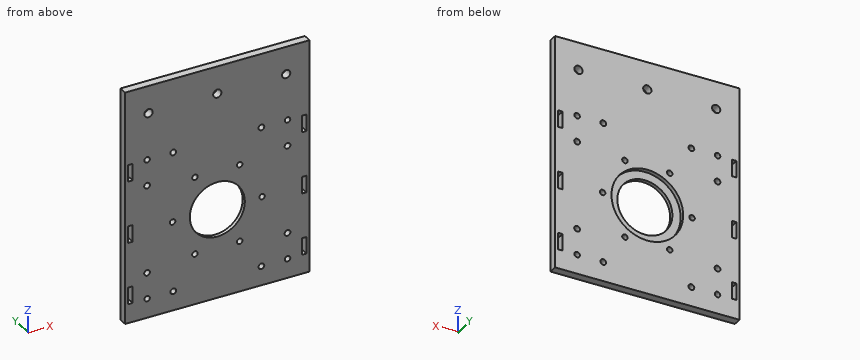
from build123d import *

# Parameters (mm, degrees)
SKETCH15_W          = 130
SKETCH15_H          = 130
SKETCH15_R          = 20
SKETCH15_R_2        = 2
BOSS_EXTRUDE1_DEPTH = 6
SKETCH16_R          = 26.05
CUT_EXTRUDE6_DEPTH  = 3.2
SKETCH17_R          = 2
CUT_EXTRUDE7_DEPTH  = 7
SKETCH18_W          = 130
SKETCH18_H          = 40
SKETCH18_R          = 3
BOSS_EXTRUDE2_DEPTH = 6
SKETCH21_W          = 2
SKETCH21_H          = 170
BOSS_EXTRUDE3_DEPTH = 6
SKETCH20_W          = 3.2
SKETCH20_H          = 12.2
CUT_EXTRUDE8_DEPTH  = 10


with BuildPart() as part:
    # Sketch15 → Boss-Extrude1 (new body)
    with BuildSketch(Plane(origin=(0, 0, 0), x_dir=(1, 0, 0), z_dir=(0, 1, 0))):
        Rectangle(SKETCH15_W, SKETCH15_H)
        Circle(SKETCH15_R, mode=Mode.SUBTRACT)
        with Locations((32.5, 0)):
            Circle(SKETCH15_R_2, mode=Mode.SUBTRACT)
        with Locations((16.25, -28.145825623)):
            Circle(SKETCH15_R_2, mode=Mode.SUBTRACT)
        with Locations((-16.25, -28.145825623)):
            Circle(SKETCH15_R_2, mode=Mode.SUBTRACT)
        with Locations((-32.5, 0)):
            Circle(SKETCH15_R_2, mode=Mode.SUBTRACT)
        with Locations((-16.25, 28.145825623)):
            Circle(SKETCH15_R_2, mode=Mode.SUBTRACT)
        with Locations((16.25, 28.145825623)):
            Circle(SKETCH15_R_2, mode=Mode.SUBTRACT)
    extrude(amount=BOSS_EXTRUDE1_DEPTH)

    # Sketch16 → Cut-Extrude6 (cut)
    with BuildSketch(Plane(origin=(0, 6, 0), x_dir=(1, 0, 0), z_dir=(0, 1, 0))):
        Circle(SKETCH16_R)
    extrude(amount=-CUT_EXTRUDE6_DEPTH, mode=Mode.SUBTRACT)

    # Sketch17 → Cut-Extrude7 (cut, through all)
    with BuildSketch(Plane.XZ):
        with Locations((-51, 51)):
            Circle(SKETCH17_R)
        with BuildLine():
            ThreePointArc((-31.999, 53.1), (-29.899, 51), (-31.999, 48.9))
            Line((-31.999, 48.9), (-32, 48.9))
            ThreePointArc((-32, 48.9), (-34.1, 51), (-32, 53.1))
            Line((-32, 53.1), (-31.999, 53.1))
        make_face()
        with BuildLine():
            Line((-53.1, 32), (-53.1, 31.999))
            ThreePointArc((-53.1, 31.999), (-51, 29.899), (-48.9, 31.999))
            Line((-48.9, 31.999), (-48.9, 32))
            ThreePointArc((-48.9, 32), (-51, 34.1), (-53.1, 32))
        make_face()
        with Locations((51, 51)):
            Circle(SKETCH17_R)
        with BuildLine():
            ThreePointArc((53.1, 31.999), (51, 29.899), (48.9, 31.999))
            Line((48.9, 31.999), (48.9, 32))
            ThreePointArc((48.9, 32), (51, 34.1), (53.1, 32))
            Line((53.1, 32), (53.1, 31.999))
        make_face()
        with Locations((51, -51)):
            Circle(SKETCH17_R)
        with BuildLine():
            Line((53.1, -32), (53.1, -31.999))
            ThreePointArc((53.1, -31.999), (51, -29.899), (48.9, -31.999))
            Line((48.9, -31.999), (48.9, -32))
            ThreePointArc((48.9, -32), (51, -34.1), (53.1, -32))
        make_face()
        with BuildLine():
            ThreePointArc((31.999, -53.1), (29.899, -51), (31.999, -48.9))
            Line((31.999, -48.9), (32, -48.9))
            ThreePointArc((32, -48.9), (34.1, -51), (32, -53.1))
            Line((32, -53.1), (31.999, -53.1))
        make_face()
        with BuildLine():
            ThreePointArc((-32, -53.1), (-34.1, -51), (-32, -48.9))
            Line((-32, -48.9), (-31.999, -48.9))
            ThreePointArc((-31.999, -48.9), (-29.899, -51), (-31.999, -53.1))
            Line((-31.999, -53.1), (-32, -53.1))
        make_face()
        with Locations((-51, -51)):
            Circle(SKETCH17_R)
        with BuildLine():
            Line((-53.1, -32), (-53.1, -31.999))
            ThreePointArc((-53.1, -31.999), (-51, -29.899), (-48.9, -31.999))
            Line((-48.9, -31.999), (-48.9, -32))
            ThreePointArc((-48.9, -32), (-51, -34.1), (-53.1, -32))
        make_face()
        with BuildLine():
            ThreePointArc((32, 53.1), (34.1, 51), (32, 48.9))
            Line((32, 48.9), (31.999, 48.9))
            ThreePointArc((31.999, 48.9), (29.899, 51), (31.999, 53.1))
            Line((31.999, 53.1), (32, 53.1))
        make_face()
    extrude(amount=-CUT_EXTRUDE7_DEPTH, mode=Mode.SUBTRACT)

    # Sketch18 → Boss-Extrude2 (add)
    with BuildSketch(Plane(origin=(0, 6, 0), x_dir=(1, 0, 0), z_dir=(0, 1, 0))):
        with Locations((0, -85)):
            Rectangle(SKETCH18_W, SKETCH18_H)
        with Locations((50, -85)):
            Circle(SKETCH18_R, mode=Mode.SUBTRACT)
        with Locations((0, -85)):
            Circle(SKETCH18_R, mode=Mode.SUBTRACT)
        with Locations((-50, -85)):
            Circle(SKETCH18_R, mode=Mode.SUBTRACT)
    extrude(amount=-BOSS_EXTRUDE2_DEPTH)

    # Sketch21 → Boss-Extrude3 (add)
    with BuildSketch(Plane(origin=(0, 6, 0), x_dir=(1, 0, 0), z_dir=(0, 1, 0))):
        with Locations((-66, -20)):
            Rectangle(SKETCH21_W, SKETCH21_H)
        with Locations((66, -20)):
            Rectangle(SKETCH21_W, SKETCH21_H)
    extrude(amount=-BOSS_EXTRUDE3_DEPTH)

    # Sketch20 → Cut-Extrude8 (cut)
    with BuildSketch(Plane(origin=(0, 6, 0), x_dir=(1, 0, 0), z_dir=(0, 1, 0))):
        with Locations((-63.1, 45)):
            Rectangle(SKETCH20_W, SKETCH20_H)
        with Locations((-63.1, 0)):
            Rectangle(SKETCH20_W, SKETCH20_H)
        with Locations((-63.1, -45)):
            Rectangle(SKETCH20_W, SKETCH20_H)
        with Locations((63.1, -45)):
            Rectangle(SKETCH20_W, SKETCH20_H)
        with Locations((63.1, 0)):
            Rectangle(SKETCH20_W, SKETCH20_H)
        with Locations((63.1, 45)):
            Rectangle(SKETCH20_W, SKETCH20_H)
    extrude(amount=-CUT_EXTRUDE8_DEPTH, mode=Mode.SUBTRACT)


solid = part.part
Could you check a few things on this model? Use its own coordinates, in mm. Coordinates: 2 decimals unless noted, no trailing zeros. Write each loop counter-clockwise with the first axis right and the second up, starting at its lowest first coordinate (ties: lowest second). Pieces come first, ordered by that corner, then holes. Notation, with made-up numbers: (18.25, -38) - (73.25, -38) arc R22 ccw to (73.25, -12) - close; hole circle Ø2 at (49, 42.25). An arc over 180 degrees is marked (long way). Write item = value, one per line.
1) Suppose I cut it at C-C on x = -16.25. Please give me the cut outline in (y, z).
Result set:
outline = (0, -65) - (6, -65) - (6, -30.15) - (0, -30.15) - close; (0, -26.15) - (6, -26.15) - (6, -20.36) - (2.8, -20.36) - (2.8, -11.66) - (0, -11.66) - close; (0, 11.66) - (2.8, 11.66) - (2.8, 20.36) - (6, 20.36) - (6, 26.15) - (0, 26.15) - close; (0, 30.15) - (6, 30.15) - (6, 105) - (0, 105) - close
2) Suppose I cut it at B-B on z = 85. Please give me the cut outline in (x, y).
Result set:
outline = (-67, 0) - (-53, 0) - (-53, 6) - (-67, 6) - close; (-47, 0) - (-3, 0) - (-3, 6) - (-47, 6) - close; (3, 0) - (47, 0) - (47, 6) - (3, 6) - close; (53, 0) - (67, 0) - (67, 6) - (53, 6) - close
3) Will this pin go through, and if not, where does the flat tip stop? pin 1 Ø3 at (x, z) = (16.25, 28.15) entering from +Y.
Result set:
pin_1 = through
4) Suppose I cut it at A-A on x = 0. Please give me the cut outline in (y, z), plus the area to 3 significant figures.
Result set:
outline = (0, -65) - (6, -65) - (6, -26.05) - (2.8, -26.05) - (2.8, -20) - (0, -20) - close; (0, 20) - (2.8, 20) - (2.8, 26.05) - (6, 26.05) - (6, 82) - (0, 82) - close; (0, 88) - (6, 88) - (6, 105) - (0, 105) - close
area = 705 mm2
5) Suppose I cut it at D-D on x = 51. Please give me the cut outline in (y, z).
Result set:
outline = (0, -65) - (6, -65) - (6, -53) - (0, -53) - close; (0, -49) - (6, -49) - (6, -34.1) - (0, -34.1) - close; (0, -29.9) - (6, -29.9) - (6, 29.9) - (0, 29.9) - close; (0, 34.1) - (6, 34.1) - (6, 49) - (0, 49) - close; (0, 53) - (6, 53) - (6, 82.17) - (0, 82.17) - close; (0, 87.83) - (6, 87.83) - (6, 105) - (0, 105) - close
6) Please list where these lines run through material, in increasing order: line 1 (Z direction, x = 0, y = 3.95); line 2 (X direction, y = 3.75, z = -44.5); line 3 (Z direction, x = -32.5, y = 4.45). Write a range as [from, to].
Result set:
line_1 = [-65, -26.05], [26.05, 82], [88, 105]
line_2 = [-67, -64.7], [-61.5, 61.5], [64.7, 67]
line_3 = [-65, -53.04], [-48.96, -2], [2, 48.96], [53.04, 105]
